from build123d import *

# Parameters (mm, degrees)
SKETCH1_W                      = 64
SKETCH1_H                      = 38
BASE_FLANGE1_DEPTH             = 5
EDGE_FLANGE1_STRIP_W           = 21.4732
EDGE_FLANGE1_STRIP_H           = 5
EDGE_FLANGE1_STRIP_CUT_DEPTH   = 64
EDGE_FLANGE1_STRIP_2_W         = 21.4732
EDGE_FLANGE1_STRIP_2_H         = 5
EDGE_FLANGE1_STRIP_CUT_2_DEPTH = 64
EDGE_FLANGE1_DEPTH             = 64
EDGE_FLANGE1_BEND_DEPTH        = 64
BREAK_CORNER1_START            = -19
BREAK_CORNER1_DEPTH            = 38
CUT_EXTRUDE1_REACH             = 64.546
SKETCH12_R                     = 4
FILLET2_R                      = 1
CHAMFER1_SIZE                  = 0.5


# Read off the part's stored shape, not the designer's step: Break-Corner1
# Sheet-metal steps are written as plain solids
with BuildPart() as part:
    # Sketch1 → Base-Flange1 (new body)
    with BuildSketch(Plane(origin=(0, 0, 0), x_dir=(1, 0, 0), z_dir=(0, 1, 0))):
        Rectangle(SKETCH1_W, SKETCH1_H)
    extrude(amount=-BASE_FLANGE1_DEPTH)

    # Edge-Flange1 strip (across the edge) → Edge-Flange1 strip cut (cut)
    with BuildSketch(Plane(origin=(-32, 0, 19), x_dir=(0, 0, -1), z_dir=(1, 0, 0))):
        with Locations((-5, -2.5)):
            Rectangle(EDGE_FLANGE1_STRIP_W, EDGE_FLANGE1_STRIP_H)
    extrude(amount=EDGE_FLANGE1_STRIP_CUT_DEPTH, mode=Mode.SUBTRACT)

    # Edge-Flange1 strip 2 (across the edge) → Edge-Flange1 strip cut 2 (cut)
    with BuildSketch(Plane(origin=(32, 0, -19), x_dir=(0, 0, 1), z_dir=(-1, 0, 0))):
        with Locations((-5, -2.5)):
            Rectangle(EDGE_FLANGE1_STRIP_2_W, EDGE_FLANGE1_STRIP_2_H)
    extrude(amount=EDGE_FLANGE1_STRIP_CUT_2_DEPTH, mode=Mode.SUBTRACT)

    # Edge-Flange1 section (across the edge) → Edge-Flange1 (add)
    with BuildSketch(Plane(origin=(-32, 0, 19), x_dir=(0, 0, -1), z_dir=(1, 0, 0))):
        with BuildLine():
            Line((0, 0.7366), (0, 38))
            Line((0, 38), (5, 38))
            Line((5, 38), (5, 0.7366))
            ThreePointArc((5, 0.7366), (5.215745145, 0.215745145), (5.7366, 0))
            Line((5.7366, 0), (5.7366, -5))
            ThreePointArc((5.7366, -5), (1.680211239, -3.319788761), (0, 0.7366))
        make_face()
    extrude(amount=EDGE_FLANGE1_DEPTH)

    # Edge-Flange1 section 2 (across the edge) → Edge-Flange1 bend (add)
    with BuildSketch(Plane(origin=(32, 0, -19), x_dir=(0, 0, 1), z_dir=(-1, 0, 0))):
        with BuildLine():
            Line((0, 0.7366), (0, 38))
            Line((0, 38), (5, 38))
            Line((5, 38), (5, 0.7366))
            ThreePointArc((5, 0.7366), (5.215745145, 0.215745145), (5.7366, 0))
            Line((5.7366, 0), (5.7366, -5))
            ThreePointArc((5.7366, -5), (1.680211239, -3.319788761), (0, 0.7366))
        make_face()
    extrude(amount=EDGE_FLANGE1_BEND_DEPTH)

    # Break-Corner1 outline → Break-Corner1 (cut)
    with BuildSketch(Plane.XY.offset(BREAK_CORNER1_START)):
        Polygon((-32, 38), (-32, 31), (-25, 38), align=None)
        Polygon((32, 38), (25, 38), (32, 31), align=None)
    extrude(amount=BREAK_CORNER1_DEPTH, mode=Mode.SUBTRACT)

    # Cut-Extrude1: up to this face of the body (flat: up to its plane)
    cut_extrude1_end = Plane(part.part.faces().sort_by_distance((0, 19.026404173, -19))[0])
    # Sketch12 → Cut-Extrude1 (cut, up to the picked face)
    with BuildSketch(Plane.XY.offset(19), mode=Mode.PRIVATE) as cut_extrude1_sk1:
        with Locations((-13.25, 22)):
            Circle(SKETCH12_R)
    cut_extrude1_tool1 = split(extrude(cut_extrude1_sk1.sketch, amount=-CUT_EXTRUDE1_REACH, mode=Mode.PRIVATE), bisect_by=cut_extrude1_end, keep=Keep.BOTH, mode=Mode.PRIVATE)
    # Sketch12 → Cut-Extrude1 (cut, up to the picked face)
    with BuildSketch(Plane.XY.offset(19), mode=Mode.PRIVATE) as cut_extrude1_sk2:
        with Locations((13.25, 22)):
            Circle(SKETCH12_R)
    cut_extrude1_tool2 = split(extrude(cut_extrude1_sk2.sketch, amount=-CUT_EXTRUDE1_REACH, mode=Mode.PRIVATE), bisect_by=cut_extrude1_end, keep=Keep.BOTH, mode=Mode.PRIVATE)
    add(cut_extrude1_tool1.solids().sort_by(Axis((-13.25, 22, 19), (0, 0, -1)))[0], mode=Mode.SUBTRACT)
    add(cut_extrude1_tool2.solids().sort_by(Axis((13.25, 22, 19), (0, 0, -1)))[0], mode=Mode.SUBTRACT)

    # Fillet2
    fillet2_edges = [part.edges().sort_by_distance(p)[0] for p in [
        (-28.5, 34.5, 14),
        (-25, 38, 16.5),
        (-28.5, 34.5, 19),
        (32, 0, 0),
        (32, -5, 0),
        (-32, 0, 0),
        (-32, -5, 0),
        (-32, -3.319788761, 17.319788761),
        (32, -3.319788761, 17.319788761),
        (-32, 0.215745145, 13.784254855),
        (32, 0.215745145, 13.784254855),
        (32, 15.8683, 14),
        (32, 15.8683, 19),
        (32, -3.319788761, -17.319788761),
        (-32, -3.319788761, -17.319788761),
        (32, 0.215745145, -13.784254855),
        (-32, 0.215745145, -13.784254855),
        (-32, 15.8683, -14),
        (-32, 15.8683, -19),
        (0, 38, -14),
        (0, 38, -19),
        (-25, 38, -16.5),
        (-28.5, 34.5, -14),
        (-32, 31, -16.5),
        (-28.5, 34.5, -19),
        (32, 15.8683, -19),
        (32, 15.8683, -14),
        (32, 31, -16.5),
        (28.5, 34.5, -14),
        (25, 38, -16.5),
        (28.5, 34.5, -19),
        (0, 38, 14),
        (0, 38, 19),
        (25, 38, 16.5),
        (28.5, 34.5, 14),
        (32, 31, 16.5),
        (28.5, 34.5, 19),
        (-32, 15.8683, 19),
        (-32, 15.8683, 14),
        (-32, 31, 16.5),
    ]]
    fillet(fillet2_edges, radius=FILLET2_R)

    # Chamfer1
    chamfer1_edges = [part.edges().sort_by_distance(p)[0] for p in [
        (-17.25, 22, -14),
        (-17.25, 22, 14),
        (-17.25, 22, 19),
        (-17.25, 22, -19),
        (9.25, 22, -14),
        (9.25, 22, 14),
        (9.25, 22, 19),
        (9.25, 22, -19),
    ]]
    chamfer(chamfer1_edges, length=CHAMFER1_SIZE)


solid = part.part
Geometry: final body of the model. Coordinates: model frame, mm. A direction names the side the tool comes from. Round coordinates to 2 decimals unless told otherwise and drop trailing zeros. Write each loop counter-clockwise with the first axis right and the second up, starting at its lowest first coordinate (ties: lowest second). Pieces come first, ordered by that corner, then holes. Notation, with made-up numbers: M -28.5,70 L 6.5,70 A15 ccw 6.5,81 Z; hole C 28.5,18.25 d4. An arc over 180 degrees is marked long. Write item = value, one per line.
Item 1: Material intervals for line 1 along Z through (x, y) = (-26, 15.5); line 2 along Y through (x, z) = (-18.5, 2.5); line 3 along Y through (x, z) = (-13.25, 16.5), sorted ascending. Write a range as [from, to].
Findings:
line_1 = [-19, -14], [14, 19]
line_2 = [-5, 0]
line_3 = [-4, 18], [26, 38]
Item 2: Access query for faces 1 (the face through (0, 19, -14)), 2 (the face through (28.332, 34.242, 18.715)), 3 (the face through (28.343, 34.253, 14.301)). Directions: +Z, -Z, +X, -X, +Y, -Y. A direction counts if a zero-diameter tool reaches every point of the face in a straight line with its end or side. Return the directions, or none.
Findings:
face_1 = +X, -X, +Y
face_2 = +Z, +X, +Y
face_3 = +X, +Y
Item 3: Section query A-A on y = 29.5. Return loops of the section in (x, z), then the cut area to 3 significant figures.
Findings:
outline = M -32,-18 A1 ccw -31,-19 L 31,-19 A1 ccw 32,-18 L 32,-15 A1 ccw 31,-14 L -31,-14 A1 ccw -32,-15 Z; M -32,15 A1 ccw -31,14 L 31,14 A1 ccw 32,15 L 32,18 A1 ccw 31,19 L -31,19 A1 ccw -32,18 Z
area = 638 mm^2
Item 4: Section query B-B on x = -13.25. State how many separate pieces and enclosed holes the cut face has, then the cut area to 3 significant figures.
Findings:
separate_pieces = 3
enclosed_holes = 0
area = 474 mm^2
Item 5: Pull-direction query (Z, two-part tool) for faces 4 (the face through (-28.242, 34.332, 18.715)), 5 (the face through (-28.242, 34.332, -18.715)), 6 (the face through (-28.242, 34.332, 14.285)); classes: pulls with the +Z half, pulls with the -Z half, needs draft (parallel to the pull), parting line crosses it, or undercut.
Findings:
face_4 = pulls with the +Z half
face_5 = pulls with the -Z half
face_6 = undercut
Item 6: Section query D-D on x = 18.5. Return loops of the section in (y, z).
Findings:
outline = M -5,-13.26 A5.74 ccw 0.74,-19 L 37,-19 A1 ccw 38,-18 L 38,-15 A1 ccw 37,-14 L 0.74,-14 A0.74 cw 0,-13.26 L 0,13.26 A0.74 cw 0.74,14 L 37,14 A1 ccw 38,15 L 38,18 A1 ccw 37,19 L 0.74,19 A5.74 ccw -5,13.26 Z
Item 7: Section query C-C on z = 9. Return loops of the section in (x, y), then the cut area to 3 significant figures.
Findings:
outline = M -32,-4 A1 ccw -31,-5 L 31,-5 A1 ccw 32,-4 L 32,-1 A1 ccw 31,0 L -31,0 A1 ccw -32,-1 Z
area = 319 mm^2
